Design review of the part shown in the three views and the two pictorial views. Dimensions are in mm from the part's minimum x, y and z. Coordinates: 2 decimals unless noted, no trailing zeros. Write each loop counter-clockwise with the first axis right and the second up, starting at its lowest first coordinate (ties: lowest second). Pieces come first, ordered by that corner, then holes. Notation, with made-up numbers: M 85.5,77 L 124.5,77 A16 cw 124.5,103 Z; hole C 60,44 d3. An arc over 180 degrees is marked long. Answer as a JSON object with one key per item and string values.
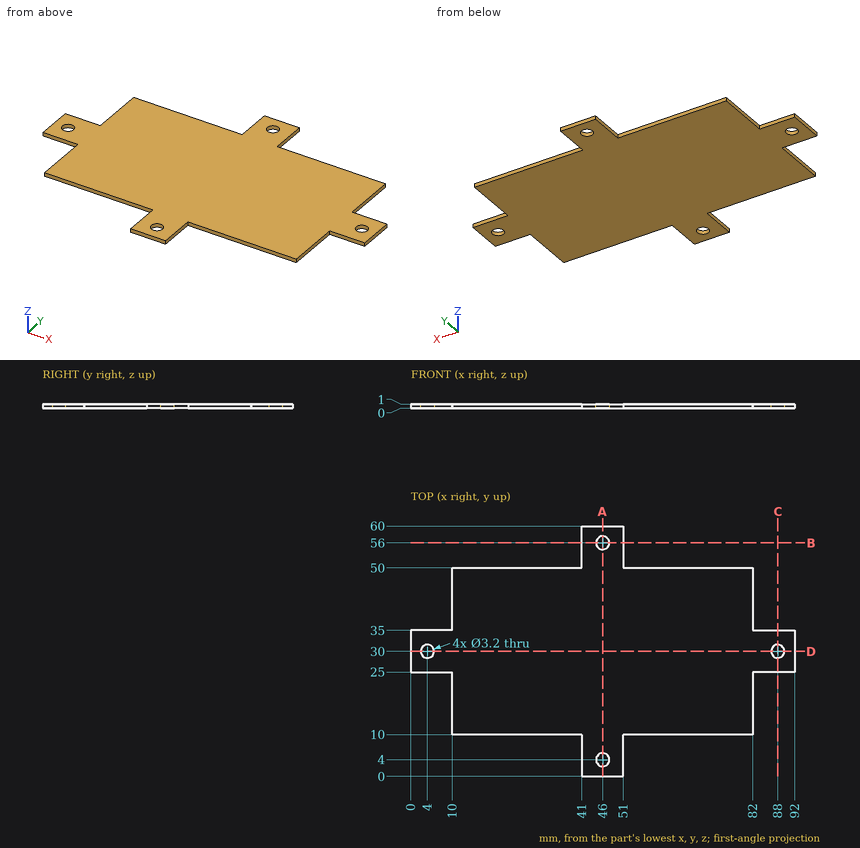
(1) Add section D-D on y = 30. Give the boundary of the cut face in (x, z).
Results list:
{"outline": "M 0,0 L 2.4,0 L 2.4,1 L 0,1 Z; M 5.6,0 L 86.4,0 L 86.4,1 L 5.6,1 Z; M 89.6,0 L 92,0 L 92,1 L 89.6,1 Z"}
(2) Add section B-B on y = 56. Give the boundary of the cut face in (x, z), and give its area (3 significant figures).
Results list:
{"outline": "M 41,0 L 44.4,0 L 44.4,1 L 41,1 Z; M 47.6,0 L 51,0 L 51,1 L 47.6,1 Z", "area": "6.80 mm²"}
(3) For pin 1 Ø1.9 at (x, y) = (4, 30) entering from +Z; pin 2 Ø0.5 at (y, z) = (3, 0.5) entering from -X; pin 3 Ø0.5 at (x, z) = (2.5, 0.5) entering from -Y; pin 4 Ø0.5 at (y, z) = (45.5, 0.5) entering from +X, all flat-tipped, find the tip position at first contact; note any pin that passes through.
Results list:
{"pin 1": "through", "pin 2": "x = 41", "pin 3": "y = 25", "pin 4": "x = 82"}
(4) Add section C-C on x = 88. Give the boundary of the cut face in (y, z), and give its area (3 significant figures).
Results list:
{"outline": "M 25,0 L 28.4,0 L 28.4,1 L 25,1 Z; M 31.6,0 L 35,0 L 35,1 L 31.6,1 Z", "area": "6.80 mm²"}
(5) Add section A-A on x = 46. Give the boundary of the cut face in (y, z), and give its area (3 significant figures).
Results list:
{"outline": "M 0,0 L 2.4,0 L 2.4,1 L 0,1 Z; M 5.6,0 L 54.4,0 L 54.4,1 L 5.6,1 Z; M 57.6,0 L 60,0 L 60,1 L 57.6,1 Z", "area": "53.6 mm²"}
(6) Wall thickness on line 1 along Y through (x, z) = (46, 0.6); line 2 along Y through (x, z) = (88, 0.8); line 3 along Y through (x, z) = (9, 0.6): over which ranges is each line inside the solid? List them lowest first. Write a range as from..to.
Results list:
{"line 1": "0..2.4, 5.6..54.4, 57.6..60", "line 2": "25..28.4, 31.6..35", "line 3": "25..35"}
